Verification items for the finished model (mm, model axes). A direction names the side the tool comes from. Round coordinates to 2 decimals unless told otherwise and drop trailing zeros. Order: outer loops, then holes, each group sorted by start corner. A loop starts at its lowest first (then second) coordinate and runs counter-clockwise, first axis right, second up. Notation, with made-up numbers: M 84,61 L 135,61 A7 ccw 135,72 Z; hole C 41.5,70 d8. An arc over 180 degrees is marked long. Answer as a JSON object with one key per item and string values. Group by question number.
```python
from build123d import *

# Parameters (mm, degrees)
SKETCH1_W           = 76.2
SKETCH1_H           = 31.75
BOSS_EXTRUDE1_DEPTH = 3.175
SKETCH2_R           = 1.27
SKETCH2_W           = 3.175
SKETCH2_H           = 7.62
CUT_EXTRUDE1_DEPTH  = 3.175


with BuildPart() as part:
    # Sketch1 → Boss-Extrude1 (new body)
    with BuildSketch(Plane(origin=(0, 0, 0), x_dir=(1, 0, 0), z_dir=(0, 1, 0))):
        Rectangle(SKETCH1_W, SKETCH1_H)
    extrude(amount=BOSS_EXTRUDE1_DEPTH)

    # Sketch2 → Cut-Extrude1 (cut)
    with BuildSketch(Plane(origin=(0, 3.175, 0), x_dir=(1, 0, 0), z_dir=(0, 1, 0))):
        with Locations(Location((-14.280312521, 0, 0), (0, 0, 270))):
            Circle(SKETCH2_R)
        with Locations(Location((22.719687479, 0, 0), (0, 0, 270))):
            Circle(SKETCH2_R)
        with Locations((-36.5125, 12.065)):
            Rectangle(SKETCH2_W, SKETCH2_H)
        with Locations((-36.5125, -12.065)):
            Rectangle(SKETCH2_W, SKETCH2_H)
    extrude(amount=-CUT_EXTRUDE1_DEPTH, mode=Mode.SUBTRACT)


solid = part.part
```
Q1. Thickness scan on line 1 (X direction, y = 1.4, z = 0); line 2 (X direction, y = 0.9, z = 0.5); line 3 (X direction, y = 2.6, z = -11) (3 decimals). Record the ranges inside material, lowest first. Write a range as from..to.
Q2. Gauge pin test, flat end, axial feed: pin 1 Ø1.6 at (y, z) = (2, 13.5) entering from -X (3 decimals). Record the tip position at first contact, or that the pin passes through.
Q3. Tool access check on faces 4 (the face through (-34.925, 2, -12)), 5 (the face through (-34.925, 2, 12)), 6 (the face through (-1, 0, 0)). Record the directions out of +Z, -Z, +X, -X, +Y, -Y that give a thin tool (end or side, any length) a straight path to the whole face; none if there is none.
Q4. Cross-section at C-C, the plane z = 10. Record the cut outline in (x, y) (3 decimals).
Q5. Cross-section at A-A, the plane z = 0. Record the cut outline in (x, y) (3 decimals).
Q6. Cross-section at B-B, the plane y = 2. Record the cut outline in (x, z) (3 decimals), then the cut area to 3 significant figures.
Q7. Release check for a two-part mould opening along X. For faces 1 (the face through (23.98, 1.61, -0.17)), 2 (the face through (-38.1, 2, 0)), 3 (the face through (-37, 2, 8.255)) record: released by +X, released by -X, zero draft, split by the parting line, or undercut.
Conclusion:
{
 "1": {"line 1": "-38.1..-15.55, -13.01..21.45, 23.99..38.1", "line 2": "-38.1..-15.45, -13.11..21.55, 23.89..38.1", "line 3": "-34.925..38.1"},
 "2": {"pin 1": "x = -34.925"},
 "3": {"face 4": "-Z, -X, +Y, -Y", "face 5": "+Z, -X, +Y, -Y", "face 6": "+Z, -Z, +X, -X, -Y"},
 "4": {"outline": "M -34.925,0 L 38.1,0 L 38.1,3.175 L -34.925,3.175 Z"},
 "5": {"outline": "M -38.1,0 L -15.55,0 L -15.55,3.175 L -38.1,3.175 Z; M -13.01,0 L 21.45,0 L 21.45,3.175 L -13.01,3.175 Z; M 23.99,0 L 38.1,0 L 38.1,3.175 L 23.99,3.175 Z"},
 "6": {"outline": "M -38.1,-8.255 L -34.925,-8.255 L -34.925,-15.875 L 38.1,-15.875 L 38.1,15.875 L -34.925,15.875 L -34.925,8.255 L -38.1,8.255 Z; hole C -14.28,0 d2.54; hole C 22.72,0 d2.54", "area": "2,360 mm2"},
 "7": {"face 1": "undercut", "face 2": "released by -X", "face 3": "zero draft"}
}
